from build123d import *

# Parameters (mm, degrees)
SKETCH2_W             = 17.554431489
SKETCH2_H             = 1.95
BOSS_EXTRUDE1_DEPTH   = 8.75
BOSS_EXTRUDE1_2_DEPTH = 8.75
CUT_EXTRUDE1_DEPTH    = 26.518349076
SKETCH4_W             = 22.027215745
SKETCH4_H             = 12.505427167
BOSS_EXTRUDE2_DEPTH   = 32
SKETCH5_R             = 1.5
CUT_EXTRUDE2_DEPTH    = 12
SKETCH6_W             = 22.027215745
SKETCH6_H             = 12.505427167
SKETCH6_W_2           = 17.554431489
SKETCH6_H_2           = 1.95
CUT_EXTRUDE3_DEPTH    = 2.5
SKETCH7_R             = 1.5
CUT_EXTRUDE4_DEPTH    = 13
SKETCH8_R             = 1.5
CUT_EXTRUDE5_DEPTH    = 34
FILLET3_R             = 1
SKETCH9_W             = 22.010837792
SKETCH9_H             = 2.932484208
SKETCH9_H_2           = 2.729697333
CUT_EXTRUDE6_DEPTH    = 11
SKETCH10_W            = 18.490355351
SKETCH10_H            = 2.932484208
SKETCH10_H_2          = 2.729697333
CUT_EXTRUDE7_DEPTH    = 5


with BuildPart() as part:
    # Sketch2 → Boss-Extrude1 (new body)
    with BuildSketch(Plane.XY):
        with Locations((-13.228930986, -27.845183414)):
            Rectangle(SKETCH2_W, SKETCH2_H)
    extrude(amount=BOSS_EXTRUDE1_DEPTH)


with BuildPart() as body_2:
    # Sketch2 → Boss-Extrude1 2 (new body)
    with BuildSketch(Plane.XY):
        with Locations((-13.228930986, -20.289756247)):
            Rectangle(SKETCH2_W, SKETCH2_H)
    extrude(amount=BOSS_EXTRUDE1_2_DEPTH)


with BuildPart() as cut_extrude1_tool:
    # Sketch3 → Cut-Extrude1 (new, through all)
    with BuildSketch(Plane(origin=(0, -19.314756247, 0), x_dir=(1, 0, 0), z_dir=(0, 1, 0))):
        with BuildLine():
            ThreePointArc((-13.228930986, -8.75), (-7.041746651, -6.187184335), (-4.478930986, 0))
            add(Edge.make_bspline(
                [(-4.478930986, 0), (1.138349918, -4.151657709), (-4.451715242, -8.75)],
                knots=[0, 0, 0, 1, 1, 1], degree=2))
            add(Edge.make_bspline(
                [(-22.006146731, -8.75), (-13.228930986, -12.473510392), (-4.451715242, -8.75)],
                knots=[0, 0, 0, 1, 1, 1], degree=2))
            add(Edge.make_bspline(
                [(-21.978930986, 0), (-25.926969228, -4.242865138), (-22.006146731, -8.75)],
                knots=[0, 0, 0, 1, 1, 1], degree=2))
            ThreePointArc((-21.978930986, 0), (-19.416115322, -6.187184335), (-13.228930986, -8.75))
        make_face()
    extrude(amount=-CUT_EXTRUDE1_DEPTH)


with BuildPart() as part_1:
    add(part.part)

    # Cut-Extrude1: cut by cut_extrude1_tool
    add(cut_extrude1_tool.part, mode=Mode.SUBTRACT)



with BuildPart() as body_2_1:
    add(body_2.part)

    # Cut-Extrude1: cut by cut_extrude1_tool
    add(cut_extrude1_tool.part, mode=Mode.SUBTRACT)


with BuildPart() as part_2:
    add(part_1.part)

    add(body_2_1.part)  # Boss-Extrude2 merges body 2
    # Sketch4 → Boss-Extrude2 (add)
    with BuildSketch(Plane(origin=(0, 0, 0), x_dir=(-1, 0, 0), z_dir=(0, 0, -1))):
        with Locations((13.242538859, -24.067469831)):
            Rectangle(SKETCH4_W, SKETCH4_H)
    extrude(amount=BOSS_EXTRUDE2_DEPTH)

    # Sketch5 → Cut-Extrude2 (cut)
    with BuildSketch(Plane(origin=(0, -19.314756247, 0), x_dir=(1, 0, 0), z_dir=(0, 1, 0))):
        with Locations(Location((-13.228930986, -2.25, 0), (0, 0, 270))):
            Circle(SKETCH5_R)
    extrude(amount=-CUT_EXTRUDE2_DEPTH, mode=Mode.SUBTRACT)

    # Sketch6 → Cut-Extrude3 (cut)
    with BuildSketch(Plane.XY):
        with Locations((-13.242538859, -24.067469831)):
            Rectangle(SKETCH6_W, SKETCH6_H)
        with Locations((-13.228930986, -27.845183414)):
            Rectangle(SKETCH6_W_2, SKETCH6_H_2, mode=Mode.SUBTRACT)
        with Locations((-13.228930986, -20.289756247)):
            Rectangle(SKETCH6_W_2, SKETCH6_H_2, mode=Mode.SUBTRACT)
    extrude(amount=-CUT_EXTRUDE3_DEPTH, mode=Mode.SUBTRACT)

    # Sketch7 → Cut-Extrude4 (cut)
    with BuildSketch(Plane(origin=(0, -17.814756247, 0), x_dir=(1, 0, 0), z_dir=(0, 1, 0))):
        with Locations(Location((-13.242538859, 25.5, 0), (0, 0, 270))):
            Circle(SKETCH7_R)
        with BuildLine():
            Line((-24.086865874, 21.155672985), (-24.256146731, 21.155672985))
            add(Edge.make_bspline(
                [(-2.228930986, 21.155672985), (11.471530889, 27.189710441), (-11.765166974, 53.431279988), (-37.007876173, 21.523583672), (-24.256146731, 21.155672985)],
                knots=[0, 0, 0, 0, 0.52011282, 1, 1, 1, 1], degree=3))
            add(Edge.make_bspline(
                [(-3.948545621, 30.585343246), (-2.007113924, 26.093685314), (-2.228930986, 21.155672985)],
                knots=[0, 0, 0, 1, 1, 1], degree=2))
            Line((-3.948545621, 30.585343246), (-13.242538859, 32))
            ThreePointArc((-13.242538859, 32), (-20.910636028, 28.823770155), (-24.086865874, 21.155672985))
        make_face()
    extrude(amount=-CUT_EXTRUDE4_DEPTH, mode=Mode.SUBTRACT)

    # Sketch8 → Cut-Extrude5 (cut)
    with BuildSketch(Plane.XY.offset(-2.5)):
        with Locations((-18.011106811, -24.06746983)):
            Circle(SKETCH8_R)
        with Locations((-8.473970906, -24.06746983)):
            Circle(SKETCH8_R)
    extrude(amount=-CUT_EXTRUDE5_DEPTH, mode=Mode.SUBTRACT)

    # Fillet3
    # the kernel refuses this fillet: 1 mm, written as the material it takes off along each edge
    with BuildSketch(Plane(origin=(-24.256146731, -15.314756247, -2.5), x_dir=(1, 0, 0), z_dir=(0, -1, 0))) as fillet3_piece_1:
        with BuildLine():
            CenterArc((FILLET3_R, -FILLET3_R), FILLET3_R, 90, 90)
            Line((0, -FILLET3_R), (-FILLET3_R * 0.02, -FILLET3_R))
            Line((-FILLET3_R * 0.02, -FILLET3_R), (-FILLET3_R * 0.02, FILLET3_R * 0.02))
            Line((-FILLET3_R * 0.02, FILLET3_R * 0.02), (FILLET3_R, FILLET3_R * 0.02))
            Line((FILLET3_R, FILLET3_R * 0.02), (FILLET3_R, 0))
        make_face()
    extrude(amount=17.505427167, mode=Mode.SUBTRACT)
    with BuildSketch(Plane(origin=(-24.256146731, -16.423026869, -21.155672985), x_dir=(0, 0, 1), z_dir=(0, -1, 0))) as fillet3_piece_2:
        with BuildLine():
            CenterArc((0.556691751, -1), FILLET3_R, 90, 33.827317624)
            Line((0, -0.169280857), (-0.011133835, -0.152666474))
            ThreePointArc((-0.011133835, -0.152666474), (-0.02, -0.084640429), (-0.02, 0))
            Line((-0.02, 0), (0, 0.02))
            Line((0, 0.02), (0.556691751, 0.02))
            Line((0.556691751, 0.02), (0.556691751, 0))
        make_face()
    extrude(amount=15.288885922, mode=Mode.SUBTRACT)
    with BuildSketch(Plane(origin=(-2.228930986, -32.820183414, -2.5), x_dir=(0, 0, -1), z_dir=(0, 1, 0))) as fillet3_piece_3:
        with BuildLine():
            CenterArc((FILLET3_R, FILLET3_R), FILLET3_R, 180, 90)
            Line((0, FILLET3_R), (-FILLET3_R * 0.02, FILLET3_R))
            Line((-FILLET3_R * 0.02, FILLET3_R), (-FILLET3_R * 0.02, -FILLET3_R * 0.02))
            Line((-FILLET3_R * 0.02, -FILLET3_R * 0.02), (FILLET3_R, -FILLET3_R * 0.02))
            Line((FILLET3_R, -FILLET3_R * 0.02), (FILLET3_R, 0))
        make_face()
    extrude(amount=17.505427167, mode=Mode.SUBTRACT)
    with BuildSketch(Plane(origin=(-3.948545621, -16.375444783, -30.585343246), x_dir=(-0.9886132451058307, 0, -0.1504787413600958), z_dir=(0, -1, 0))) as fillet3_piece_4:
        with BuildLine():
            CenterArc((0.562435527, -1), FILLET3_R, 90, 59.471323616)
            Line((-0.298939504, -0.492030458), (-0.316167005, -0.481871067))
            ThreePointArc((-0.316167005, -0.481871067), (-0.168173949, -0.234650824), (-0.016955383, 0.010607308))
            Line((-0.016955383, 0.010607308), (0, 0.02))
            Line((0, 0.02), (0.562435527, 0.02))
            Line((0.562435527, 0.02), (0.562435527, 0))
        make_face()
    extrude(amount=15.384050094, mode=Mode.SUBTRACT)

    # Sketch9 → Cut-Extrude6 (cut)
    with BuildSketch(Plane.XY.offset(-32.5)):
        with Locations((-13.24253886, -20.332641731)):
            Rectangle(SKETCH9_W, SKETCH9_H)
        with Locations((-13.24253886, -27.700904501)):
            Rectangle(SKETCH9_W, SKETCH9_H_2)
    extrude(amount=CUT_EXTRUDE6_DEPTH, mode=Mode.SUBTRACT)

    # Sketch10 → Cut-Extrude7 (cut)
    with BuildSketch(Plane(origin=(0, 0, -21.5), x_dir=(-1, 0, 0), z_dir=(0, 0, -1))):
        with Locations((13.054523996, -20.332641731)):
            Rectangle(SKETCH10_W, SKETCH10_H)
        with Locations((13.054523996, -27.700904501)):
            Rectangle(SKETCH10_W, SKETCH10_H_2)
    extrude(amount=-CUT_EXTRUDE7_DEPTH, mode=Mode.SUBTRACT)


solid = part_2.part
Design review of the part built by this model. Coordinates are the model's own, in mm. A direction names the side the tool comes from. Round coordinates to 2 decimals unless told otherwise and drop trailing zeros. Write each loop counter-clockwise with the first axis right and the second up, starting at its lowest first coordinate (ties: lowest second). Pieces come first, ordered by that corner, then holes. Notation, with made-up numbers: (-34.75, 54) - (-5.75, 54) arc R17 cw to (-5.75, 87) - close; hole circle Ø6 at (-10.5, 77.25). An arc over 180 degrees is marked (long way). Return JSON: item names as keys, results as strings. Group by question number.
Item 1: For probe 1 along Y at (x, z) = (-11.75, -19.5); probe 2 along Y at (x, z) = (-11.75, 6); probe 3 along Y at (x, z) = (-18, -16), list the stretches that pass through material, from the lowest coordinate up. Write a range as [from, to].
Item 2: Machinability: for faces 1 (the face through (-22.006, -20, -1)), 2 (the face through (-15, -21.265, 2)), 3 (the face through (-13, -20, -16.5)), which of the approach directions +Z, -Z, +X, -X, +Y, -Y give a long, thin tool a straight path to every point of the face, cutting with its end or side? Answer none if there is none.
Item 3: The part is to be moulded in two halves that separate along Y. For faces 4 (the face through (-13.2, -18.3, -27)), 5 (the face through (-15, -19.315, 2)), 6 (the face through (-13, -26.336, -23)), say which applies: pulls with the +Y half, pulls with the -Y half, needs draft (parallel to the pull), parting line crosses it, or undercut.
Item 4: We need section B-B on x = -9. Write out the cut boundary in (y, z).
Item 5: We need section C-C on z = -25.5. Give the number of separate pieces and of enclosed holes in the cut face, and give its area (3 significant figures).
Item 6: Insertion check: P1, Ø2, axis at y = -22.5, z = 4, coming from the -X side; P2, Ø2, axis at x = -23, y = -20.5, coming from the -Z side; P3, Ø1, axis at y = -20, z = -0.5, coming from the -X side; P4, Ø1.5, axis at x = -16, y = -20.5, coming from the -Z side. Each pin has a flat end and moves straight along its axis. Give the tip position at first contact, or say it passes through.
Item 7: We need section A-A on z = 2.25. Write out the cut boundary in (x, y).
Item 8: We need section D-D on z = -10.5. Write out the cut boundary in (x, y).
Model answer:
{
 "1": {"probe 1": "y = [-30.32, -29.07], [-26.34, -21.8], [-18.87, -17.81]", "probe 2": "y = [-28.82, -26.87], [-21.26, -19.31]", "probe 3": "y = [-30.32, -25.57], [-22.57, -17.81]"},
 "2": {"face 1": "+Z, -X, +Y, -Y", "face 2": "+Z, +X, -X", "face 3": "-Z"},
 "3": {"face 4": "needs draft", "face 5": "pulls with the +Y half", "face 6": "undercut"},
 "4": {"outline": "(-30.32, -31.35) - (-29.07, -31.35) - (-29.07, -16.5) - (-26.34, -16.5) - (-26.34, -31.35) - (-25.47, -31.35) - (-25.47, -2.5) - (-26.87, -2.5) - (-26.87, 7.66) - (-28.82, 7.66) - (-28.82, -2.5) - (-30.32, -2.5) - close; (-22.66, -31.35) - (-21.8, -31.35) - (-21.8, -16.5) - (-18.87, -16.5) - (-18.87, -31.35) - (-17.81, -31.35) - (-17.81, -2.5) - (-19.31, -2.5) - (-19.31, 7.66) - (-21.26, 7.66) - (-21.26, -2.5) - (-22.66, -2.5) - close"},
 "5": {"separate pieces": "6", "enclosed holes": "2", "area": "107 mm²"},
 "6": {"P1": "passes through", "P2": "stops at z = -21.5", "P3": "stops at x = -22.01", "P4": "stops at z = -16.5"},
 "7": {"outline": "(-21.68, -28.82) - (-14.73, -28.82) - (-14.73, -26.87) - (-21.68, -26.87) - close; (-21.68, -21.26) - (-14.73, -21.26) - (-14.73, -19.31) - (-21.68, -19.31) - close; (-11.73, -28.82) - (-4.77, -28.82) - (-4.77, -26.87) - (-11.73, -26.87) - close; (-11.73, -21.26) - (-4.77, -21.26) - (-4.77, -19.31) - (-11.73, -19.31) - close"},
 "8": {"outline": "(-24.26, -30.32) - (-2.23, -30.32) - (-2.23, -17.81) - (-24.26, -17.81) - close; hole circle Ø3 at (-18.01, -24.07); hole circle Ø3 at (-8.47, -24.07)"}
}
